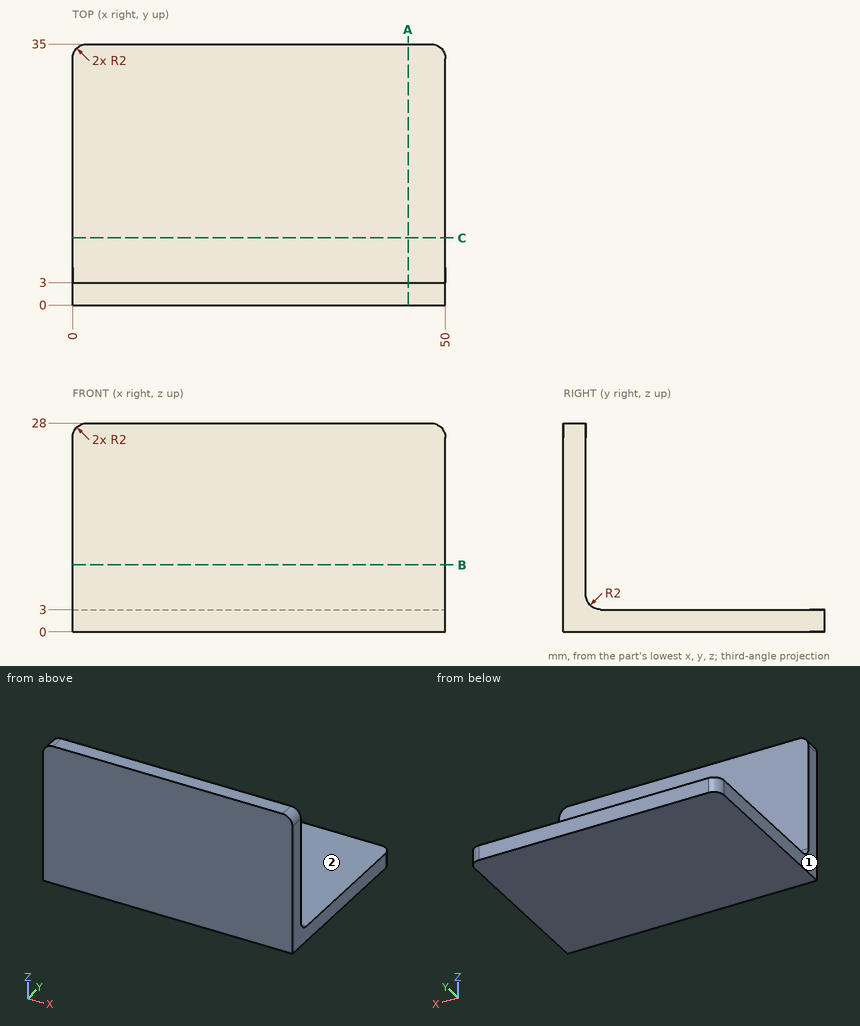
For this review, use the dimensioned drawing (mm, ordinates from the lowest corner) and the shaded views. A direction names the side the tool comes from. Coordinates: 2 decimals unless noted, no trailing zeros. Loops run counter-clockwise (first coordinate to the right, second up) from the corner with the lowest first, then second, coordinate; pieces in that order, holes last. Notation, with made-up numbers: (86.5, 63) -> (96.5, 63) arc R19 cw to (96.5, 98) -> close; hole circle Ø9 at (21, -40). An arc over 180 degrees is marked (long way). Use a Markdown table: item, result. Add a question column.
Item 1: Clearance check with flat-ended pins moving along their axes: P1, Ø12, axis at x = 9, y = 24, coming from the -Z side; P2, Ø1.5, axis at y = 28.5, z = 5.5, coming from the -X side; P3, Ø9, axis at x = 37, y = 13, coming from the +Z side; P4, Ø12, axis at x = 31, z = 25, coming from the +Y side. State where each tip first meets the part, or that it passes through.
Item 2: We need section A-A, the plane x = 45. Write out the cut boundary in (y, z), and give its area (3 significant figures).
Item 3: Wall thickness on L1, parallel to Y at x = 36.5, z = 14.75: over which ranges is the line inside the solid? List them lowest first. Write a range as from..to.
Item 4: We need section B-B, the plane z = 9. Write out the cut boundary in (x, y).
Item 5: Machinability: for the marked faces 1 and 2, which of the approach directions +Z, -Z, +X, -X, +Y, -Y give a long, thin tool a straight path to every point of the face, cutting with its end or side? Answer none if there is none.
Numbers:
| question | item | result |
|---|---|---|
| 1 | P1 | stops at z = 0 |
| 1 | P2 | passes through |
| 1 | P3 | stops at z = 3 |
| 1 | P4 | stops at y = 3 |
| 2 | outline | (0, 0) -> (35, 0) -> (35, 3) -> (5, 3) arc R2 cw to (3, 5) -> (3, 28) -> (0, 28) -> close |
| 2 | area | 181 mm^2 |
| 3 | L1 | y = 0..3 |
| 4 | outline | (0, 0) -> (50, 0) -> (50, 3) -> (0, 3) -> close |
| 5 | face 1 | +Z, -Z, -X, +Y, -Y |
| 5 | face 2 | +Z, +X, -X, +Y |
